For this review, take the finished solid that the model builds, in its own axes (mm). Face numbers are marked on the shaded views. A direction names the side the tool comes from. Coordinates: 2 decimals unless noted, no trailing zeros. Order: outer loops, then holes, each group sorted by start corner. A loop starts at its lowest first (then second) coordinate and runs counter-clockwise, first axis right, second up. Notation, with made-up numbers: (69, 2) -> (87, 2) arc R16 cw to (87, 10) -> close; hole circle Ø10 at (68, 60.5). An arc over 180 degrees is marked (long way). Write item = value, one per line. Start each with the question number.
1) Draft analysis for pull direction Y (two halves, no side actions). For the marked faces 3, 4, 5 and 6, state which applies: +Y half, -Y half, draft (parallel to the pull), parting line (faces both ways), or undercut.
2) Consider section C-C on x = -38.1. Give the boundary of the cut face in (y, z).
3) Wall thickness on probe 1 along X at (y, z) = (25.5, 14); probe 2 along Y at (x, z) = (38, 16); probe 3 along Z at (x, y) = (15, -11.5): over which ranges is each line inside the solid? List them lowest first. Write a range as [from, to].
4) Consider section A-A on z = 15.5. Give the boundary of the cut face in (x, y).
5) Insertion check: pin 1 Ø1 at (x, z) = (-7.5, 32) entering from -Y; pin 2 Ø14.5 at (x, y) = (38.1, 25.4) entering from -Z; pin 3 Ø3 at (x, z) = (-19, 59.5) entering from +Y; pin 4 Ø3 at (x, z) = (-27.5, 68) entering from +Y. Each pin has a flat end and moves straight along its axis. Give the tip position at first contact, or say it passes through.
6) Machinability: for the marked faces 1 and 2, which of the approach directions +Z, -Z, +X, -X, +Y, -Y give a long, thin tool a straight path to every point of the face, cutting with its end or side? Answer none if there is none.
7) Consider section D-D on y = 0. Give the boundary of the cut face in (x, z).
8) Consider section B-B on x = 0. Give the boundary of the cut face in (y, z), and give its area (3 significant figures).
from build123d import *

# Parameters (mm, degrees)
F0_W     = 101.6
F0_H     = 76.2
F1_DEPTH = 25.4
F2_R     = 6.35
F3_DEPTH = 25.4
F4_R     = 25.4
F5_DEPTH = 50.8
F6_W     = 61.2722363651
F6_H     = 6.35
F8_R     = 5.08


# Not quite as in the source:
# - a fillet or chamfer that OpenCascade refuses, or shapes differently, is made with other operations: its cross-section is extruded or revolved along the edge and cut away or added


with BuildPart() as f1:
    # F0 (on Top) → F1 (new body)
    with BuildSketch(Plane.XY):
        Rectangle(F0_W, F0_H)
    extrude(amount=F1_DEPTH)

    # F2 (on face) → F3 (cut, through all)
    with BuildSketch(Plane.XY.offset(25.4)):
        with Locations((-38.1, 25.4)):
            Circle(F2_R)
        with Locations((38.1, 25.4)):
            Circle(F2_R)
        with Locations((38.1, -25.4)):
            Circle(F2_R)
        with Locations((-38.1, -25.4)):
            Circle(F2_R)
    extrude(amount=-F3_DEPTH, mode=Mode.SUBTRACT)

    # F4 (on face) → F5 (join)
    with BuildSketch(Plane.XY.offset(25.4)):
        Circle(F4_R)
    extrude(amount=F5_DEPTH)

    # F6 (on Front) → F7 (revolve, cut)
    with BuildSketch(Plane.XZ):
        with Locations((-43.3361181825, 35.8842967927)):
            Rectangle(F6_W, F6_H)
    revolve(axis=Axis((0, 0, 28.4035503864), (0, 0, 1)), mode=Mode.SUBTRACT)

    # F8
    f8_edges = [f1.edges().sort_by_distance(p)[0] for p in [
        (0, -38.1, 25.4),
        (-25.4, 0, 32.709297),
        (-25.4, 0, 39.059297),
        (-25.4, 0, 76.2),
        (50.8, 0, 25.4),
        (0, 38.1, 25.4),
        (-50.8, 0, 25.4),
    ]]
    fillet(f8_edges, radius=F8_R)

    # F9: chamfer of 5.08 on 12 edges, made by hand

    # F9_s1 → F9_t2 (revolve, cut)
    with BuildSketch(Plane.XZ.offset(25.4)):
        Polygon((-26.67, 25.4), (-31.75, 20.32), (-31.75, 25.4), align=None)
    revolve(axis=Axis((-38.1, -25.4, 25.4), (0, 0, 1)), mode=Mode.SUBTRACT)

    # F9_s3 → F9_t4 (revolve, cut)
    with BuildSketch(Plane.XZ.offset(25.4)):
        Polygon((-26.67, 0), (-31.75, 5.08), (-31.75, 0), align=None)
    revolve(axis=Axis((-38.1, -25.4, 0), (0, 0, 1)), mode=Mode.SUBTRACT)

    # F9_s5 → F9_t6 (revolve, cut)
    with BuildSketch(Plane.XZ.offset(-25.4)):
        Polygon((-26.67, 25.4), (-31.75, 20.32), (-31.75, 25.4), align=None)
    revolve(axis=Axis((-38.1, 25.4, 25.4), (0, 0, 1)), mode=Mode.SUBTRACT)

    # F9_s7 → F9_t8 (revolve, cut)
    with BuildSketch(Plane.XZ.offset(-25.4)):
        Polygon((-26.67, 0), (-31.75, 5.08), (-31.75, 0), align=None)
    revolve(axis=Axis((-38.1, 25.4, 0), (0, 0, 1)), mode=Mode.SUBTRACT)

    # F9_s9 → F9_t10 (revolve, cut)
    with BuildSketch(Plane.XZ.offset(-25.4)):
        Polygon((49.53, 25.4), (44.45, 20.32), (44.45, 25.4), align=None)
    revolve(axis=Axis((38.1, 25.4, 25.4), (0, 0, 1)), mode=Mode.SUBTRACT)

    # F9_s11 → F9_t12 (revolve, cut)
    with BuildSketch(Plane.XZ.offset(-25.4)):
        Polygon((49.53, 0), (44.45, 5.08), (44.45, 0), align=None)
    revolve(axis=Axis((38.1, 25.4, 0), (0, 0, 1)), mode=Mode.SUBTRACT)

    # F9_s13 → F9_t14 (revolve, cut)
    with BuildSketch(Plane.XZ.offset(25.4)):
        Polygon((49.53, 25.4), (44.45, 20.32), (44.45, 25.4), align=None)
    revolve(axis=Axis((38.1, -25.4, 25.4), (0, 0, 1)), mode=Mode.SUBTRACT)

    # F9_s15 → F9_t16 (revolve, cut)
    with BuildSketch(Plane.XZ.offset(25.4)):
        Polygon((49.53, 0), (44.45, 5.08), (44.45, 0), align=None)
    revolve(axis=Axis((38.1, -25.4, 0), (0, 0, 1)), mode=Mode.SUBTRACT)


solid = f1.part
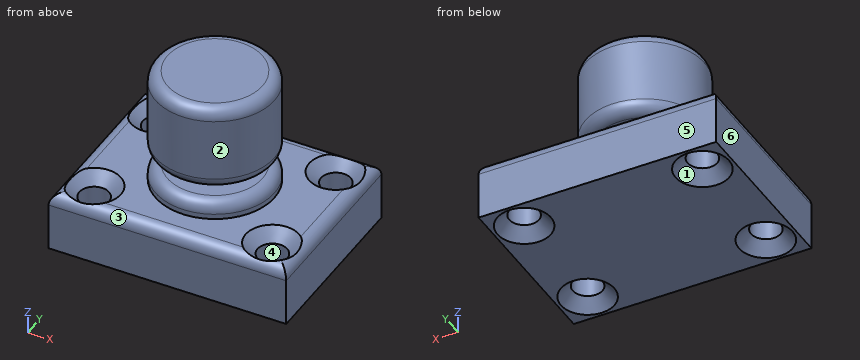
Answer sheet:
q1.face_3 = -Y half
q1.face_4 = undercut
q1.face_5 = +Y half
q1.face_6 = draft
q2.outline = (-38.1, 0) -> (-36.83, 0) -> (-31.75, 5.08) -> (-31.75, 20.32) -> (-35.92, 24.49) arc R5.08 ccw to (-38.1, 20.32) -> close; (-19.05, 5.08) -> (-13.97, 0) -> (13.97, 0) -> (19.05, 5.08) -> (19.05, 20.32) -> (13.97, 25.4) -> (-13.97, 25.4) -> (-19.05, 20.32) -> close; (31.75, 5.08) -> (36.83, 0) -> (38.1, 0) -> (38.1, 20.32) arc R5.08 ccw to (35.92, 24.49) -> (31.75, 20.32) -> close
q3.probe_1 = [-50.8, -44.45], [-31.75, 31.75], [44.45, 50.8]
q3.probe_2 = [-38.1, -31.75], [-19.05, 19.05], [31.75, 38.1]
q3.probe_3 = [0, 32.71], [39.06, 76.2]
q4.outline = (-50.8, -38.1) -> (50.8, -38.1) -> (50.8, 38.1) -> (-50.8, 38.1) -> close; hole circle Ø12.7 at (-38.1, -25.4); hole circle Ø12.7 at (-38.1, 25.4); hole circle Ø12.7 at (38.1, -25.4); hole circle Ø12.7 at (38.1, 25.4)
q5.pin_1 = -22.41
q5.pin_2 = 4.18
q5.pin_3 = 18.41
q5.pin_4 = through
q6.face_1 = -Z
q6.face_2 = +Z
q7.outline = (-50.8, 0) -> (50.8, 0) -> (50.8, 20.32) arc R5.08 ccw to (45.72, 25.4) -> (25.4, 25.4) -> (25.4, 27.63) arc R5.08 ccw to (20.32, 32.71) -> (12.7, 32.71) -> (12.7, 39.06) -> (20.32, 39.06) arc R5.08 ccw to (25.4, 44.14) -> (25.4, 71.12) arc R5.08 ccw to (20.32, 76.2) -> (-20.32, 76.2) arc R5.08 ccw to (-25.4, 71.12) -> (-25.4, 44.14) arc R5.08 ccw to (-20.32, 39.06) -> (-12.7, 39.06) -> (-12.7, 32.71) -> (-20.32, 32.71) arc R5.08 ccw to (-25.4, 27.63) -> (-25.4, 25.4) -> (-45.72, 25.4) arc R5.08 ccw to (-50.8, 20.32) -> close
q8.outline = (-38.1, 0) -> (38.1, 0) -> (38.1, 20.32) arc R5.08 ccw to (33.02, 25.4) -> (25.4, 25.4) -> (25.4, 27.63) arc R5.08 ccw to (20.32, 32.71) -> (12.7, 32.71) -> (12.7, 39.06) -> (20.32, 39.06) arc R5.08 ccw to (25.4, 44.14) -> (25.4, 71.12) arc R5.08 ccw to (20.32, 76.2) -> (-20.32, 76.2) arc R5.08 ccw to (-25.4, 71.12) -> (-25.4, 44.14) arc R5.08 ccw to (-20.32, 39.06) -> (-12.7, 39.06) -> (-12.7, 32.71) -> (-20.32, 32.71) arc R5.08 ccw to (-25.4, 27.63) -> (-25.4, 25.4) -> (-33.02, 25.4) arc R5.08 ccw to (-38.1, 20.32) -> close
q8.area = 4,310 mm2
